from build123d import *

# Parameters (mm, degrees)
EXTRUDE_1_DEPTH     = 2.5
FILLET_1_R          = 3
SKETCH_2_R          = 1.525
EXTRUDE_2_DEPTH     = 5
SKETCH_3_R          = 2
EXTRUDE_3_DEPTH     = 1
SKETCH_4_R          = 5.975
CUT_EXTRUDE_1_DEPTH = 10
EXTRUDE_4_DEPTH     = 1
SKETCH_6_R          = 4.5
CUT_EXTRUDE_2_DEPTH = 1
SKETCH_7_R          = 1
CUT_EXTRUDE_3_DEPTH = 10
SKETCH_9_R          = 16.5
CUT_EXTRUDE_4_DEPTH = 10


with BuildPart() as part:
    # 草图1 → 凸台-拉伸1 (new body)
    with BuildSketch(Plane.XY):
        Polygon((-15.588457268, -9), (15.588457268, -9), (0, 18), align=None)
        Polygon((10.392304845, -6), (0, 12), (-10.392304845, -6), align=None, mode=Mode.SUBTRACT)
        Polygon((-10.392304845, -6), (10.392304845, -6), (0, 12), align=None)
    extrude(amount=EXTRUDE_1_DEPTH)

    # 圆角1
    fillet_1_edges = [part.edges().sort_by_distance(p)[0] for p in [
        (-15.588457268, -9, 1.25),
        (0, 18, 1.25),
        (15.588457268, -9, 1.25),
    ]]
    fillet(fillet_1_edges, radius=FILLET_1_R)

    # 草图2 → 凸台-拉伸2 (add)
    with BuildSketch(Plane.XY.offset(2.5)):
        with Locations((0, 12)):
            Circle(SKETCH_2_R)
        with Locations((10.392304845, -6)):
            Circle(SKETCH_2_R)
        with Locations((-10.392304845, -6)):
            Circle(SKETCH_2_R)
    extrude(amount=EXTRUDE_2_DEPTH)

    # 草图3 → 凸台-拉伸3 (add)
    with BuildSketch(Plane.XY.offset(2.5)):
        with Locations((0, 12)):
            Circle(SKETCH_3_R)
        with Locations((10.392304845, -6)):
            Circle(SKETCH_3_R)
        with Locations((-10.392304845, -6)):
            Circle(SKETCH_3_R)
    extrude(amount=EXTRUDE_3_DEPTH)

    # 草图4 → 切除-拉伸1 (cut)
    with BuildSketch(Plane(origin=(0, 0, 0), x_dir=(-1, 0, 0), z_dir=(0, 0, -1))):
        Circle(SKETCH_4_R)
    extrude(amount=-CUT_EXTRUDE_1_DEPTH, mode=Mode.SUBTRACT)

    # 草图5 → 凸台-拉伸4 (add)
    with BuildSketch(Plane(origin=(0, 0, 0), x_dir=(-1, 0, 0), z_dir=(0, 0, -1))):
        with BuildLine():
            Line((-10.392304845, -9), (10.392304845, -9))
            ThreePointArc((10.392304845, -9), (12.990381057, -7.5), (12.990381057, -4.5))
            Line((12.990381057, -4.5), (2.598076211, 13.5))
            ThreePointArc((2.598076211, 13.5), (0, 15), (-2.598076211, 13.5))
            Line((-2.598076211, 13.5), (-12.990381057, -4.5))
            ThreePointArc((-12.990381057, -4.5), (-12.990381057, -7.5), (-10.392304845, -9))
        make_face()
    extrude(amount=EXTRUDE_4_DEPTH)

    # 草图6 → 切除-拉伸2 (cut)
    with BuildSketch(Plane.XY):
        Circle(SKETCH_6_R)
    extrude(amount=-CUT_EXTRUDE_2_DEPTH, mode=Mode.SUBTRACT)

    # 草图7 → 切除-拉伸3 (cut)
    with BuildSketch(Plane.XY.offset(2.5)):
        with Locations((0, 7.5)):
            Circle(SKETCH_7_R)
        with Locations((6.495190528, -3.75)):
            Circle(SKETCH_7_R)
        with Locations((-6.495190528, -3.75)):
            Circle(SKETCH_7_R)
    extrude(amount=-CUT_EXTRUDE_3_DEPTH, mode=Mode.SUBTRACT)

    # 草图9 → 切除-拉伸4 (cut)
    with BuildSketch(Plane.XY.offset(2.5)):
        with Locations((-20, 11.547005384)):
            Circle(SKETCH_9_R)
        with Locations((20, 11.547005384)):
            Circle(SKETCH_9_R)
        with Locations((0, -23.094010768)):
            Circle(SKETCH_9_R)
    extrude(amount=-CUT_EXTRUDE_4_DEPTH, mode=Mode.SUBTRACT)


solid = part.part
CAD build for the part. Positions are in the model's coordinates, mm. A direction names the side the tool comes from. Give positions to 0.01 mm unless a question says otherwise; leave off trailing zeros. Loops run counter-clockwise (first coordinate to the right, second up) from the corner with the lowest first, then second, coordinate; pieces in that order, holes last. Notation, with made-up numbers: M 27.25,64 L 73.25,64 A7 cw 73.25,70 Z; hole C 39,19 d8. An arc over 180 degrees is marked long. Answer in a Markdown table with one row per item. Add a question column.
Item 1: Band-saw the part on D-D on y = 11. Give the cut face in (x, z).
Item 2: Drop flat-ended pins along their axis: P1, Ø9.5, axis at x = -2.5, y = 0, coming from the +Z side; P2, Ø4, axis at y = 12, z = 6, coming from the -X side (3 decimals). Give the stop position or say it passes through.
Item 3: Band-saw the part on C-C on x = -10.75. Give the cut face in (y, z), then the cut area to 3 significant figures.
Item 4: Tool access for faces 1 (the face through (-0.13, 8.49, 0.77)), 2 (the face through (8.394, -5.912, 2.993)): list every direction of +Z, -Z, +X, -X, +Y, -Y with a clear straight run to the whole face (end or side of a thin tool).
Item 5: Band-saw the part on A-A on y = 7.5. Give the cut face in (x, z), then the cut area to 3 significant figures.
Item 6: Band-saw the part on B-B on z = 3. Give the cut face in (x, y), then the cut area to 3 significant figures.
Item 7: Probe probe 1 along Y at (x, z) = (0, 1.75) (3 decimals); probe 2 along Z at (x, y) = (-6.75, 0); probe 3 along X at (y, z) = (-6.75, 5). List the from-to ranges inside material, lowest first.
Reply:
| question | item | result |
|---|---|---|
| 1 | outline | M -3.51,-1 L 3.51,-1 L 3.51,2.5 L 1.73,2.5 L 1.73,3.5 L 1.15,3.5 L 1.15,7.5 L -1.15,7.5 L -1.15,3.5 L -1.73,3.5 L -1.73,2.5 L -3.51,2.5 Z |
| 2 | P1 | stops at z = 2.5 |
| 2 | P2 | stops at x = -1.525 |
| 3 | outline | M -8.98,-1 L -2.12,-1 L -2.12,2.5 L -4.03,2.5 L -4.03,3.5 L -4.52,3.5 L -4.52,7.5 L -7.48,7.5 L -7.48,3.5 L -7.97,3.5 L -7.97,2.5 L -8.98,2.5 Z |
| 3 | area | 39.8 mm^2 |
| 4 | face 1 | +Z, -Z |
| 4 | face 2 | +Z |
| 5 | outline | M -4,-1 L -1,-1 L -1,2.5 L -4,2.5 Z; M 1,-1 L 4,-1 L 4,2.5 L 1,2.5 Z |
| 5 | area | 21.0 mm^2 |
| 6 | outline | C -10.39,-6 d4; C 0,12 d4; C 10.39,-6 d4 |
| 6 | area | 37.7 mm^2 |
| 7 | probe 1 | y = -6.594 to -5.975, 5.975 to 6.5, 8.5 to 15 |
| 7 | probe 2 | z = -1 to 2.5 |
| 7 | probe 3 | x = -11.72 to -9.06, 9.06 to 11.72 |
